Input: dimensioned drawing with shaded views. Units: mm. Origin: part minimum x, y, z. Give positions to 0.01 mm unless a question says otherwise; leave off trailing zeros. Order: outer loops, then holes, each group sorted by start corner. A loop starts at its lowest first (then second) coordinate and runs counter-clockwise, first axis right, second up.
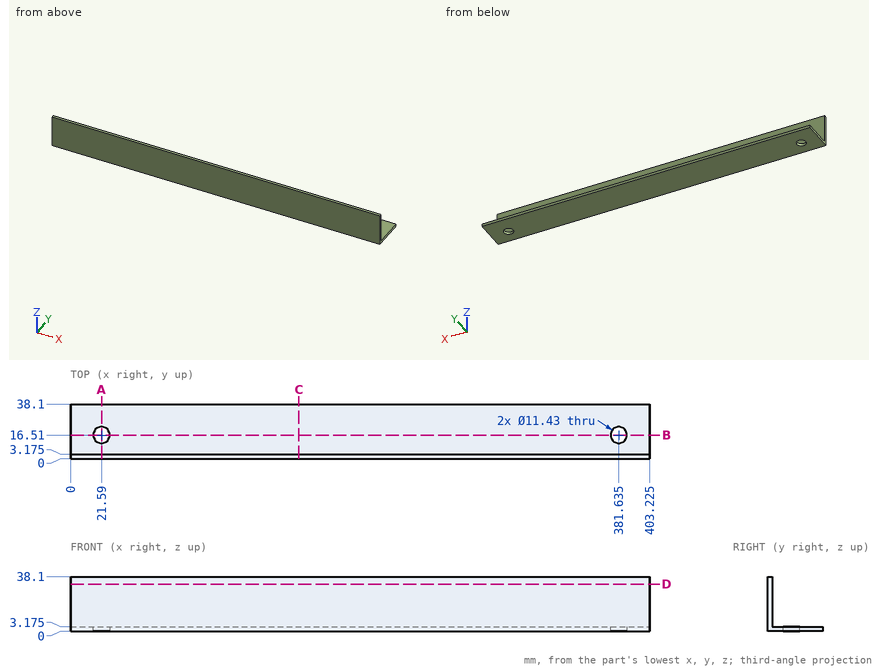
1) Section query B-B, the plane y = 16.51. Return the cut outline in (x, z) (3 decimals), and give its area (3 significant figures).
Report:
outline: (0, 0) - (15.875, 0) - (15.875, 3.175) - (0, 3.175) - close; (27.305, 0) - (375.92, 0) - (375.92, 3.175) - (27.305, 3.175) - close; (387.35, 0) - (403.225, 0) - (403.225, 3.175) - (387.35, 3.175) - close
area: 1,210 mm2
2) Section query D-D, the plane z = 33. Return the cut outline in (x, y) (3 decimals).
Report:
outline: (0, 0) - (403.225, 0) - (403.225, 3.175) - (0, 3.175) - close
3) Section query A-A, the plane x = 21.59. Return the cut outline in (y, z) (3 decimals), and give its area (3 significant figures).
Report:
outline: (0, 0) - (10.795, 0) - (10.795, 3.175) - (3.175, 3.175) - (3.175, 38.1) - (0, 38.1) - close; (22.225, 0) - (38.1, 0) - (38.1, 3.175) - (22.225, 3.175) - close
area: 196 mm2
4) Material intervals for L1, parallel to X at y = 16, z = 1 (3 decimals); L2, parallel to Y at x = 21, z = 2; L3, parallel to Y at x = 241.5, z = 25 (3 decimals), sorted ascending.
Report:
L1: x = 0 to 15.898, 27.282 to 375.943, 387.327 to 403.225
L2: y = 0 to 10.83, 22.19 to 38.1
L3: y = 0 to 3.175
5) Pin query (flat end, axial travel): pin 1 (1.5 mm diameter, centred on x = 113, z = 14, fed in from +Y) (3 decimals); pin 2 (10.5 mm diameter, centred on x = 298.5, y = 14.5, fed in from +Z) (3 decimals). Return the tip coordinate at first contact, or that it passes through.
Report:
pin 1: stops at y = 3.175
pin 2: stops at z = 3.175
6) Section query C-C, the plane x = 159. Return the cut outline in (y, z) (3 decimals).
Report:
outline: (0, 0) - (38.1, 0) - (38.1, 3.175) - (3.175, 3.175) - (3.175, 38.1) - (0, 38.1) - close
